from build123d import *

# Parameters (mm, degrees)
EXTRUDE_1_DEPTH = 2


with BuildPart() as part:
    # 草图1 → 凸台-拉伸1 (new body)
    with BuildSketch(Plane.XY):
        with BuildLine():
            Line((-56, 150), (56, 150))
            ThreePointArc((56, 150), (58.828427125, 148.828427125), (60, 146))
            Line((60, 146), (60, 144))
            ThreePointArc((60, 144), (58.828427125, 141.171572875), (56, 140))
            Line((56, 140), (8, 140))
            Line((8, 140), (8, -140))
            Line((8, -140), (56, -140))
            ThreePointArc((56, -140), (58.828427125, -141.171572875), (60, -144))
            Line((60, -144), (60, -146))
            ThreePointArc((60, -146), (58.828427125, -148.828427125), (56, -150))
            Line((56, -150), (-56, -150))
            ThreePointArc((-56, -150), (-58.828427125, -148.828427125), (-60, -146))
            Line((-60, -146), (-60, -144))
            ThreePointArc((-60, -144), (-58.828427125, -141.171572875), (-56, -140))
            Line((-56, -140), (-8, -140))
            Line((-8, -140), (-8, 140))
            Line((-8, 140), (-56, 140))
            ThreePointArc((-56, 140), (-58.828427125, 141.171572875), (-60, 144))
            Line((-60, 144), (-60, 146))
            ThreePointArc((-60, 146), (-58.828427125, 148.828427125), (-56, 150))
        make_face()
    extrude(amount=EXTRUDE_1_DEPTH)


solid = part.part
Geometry: final body of the model. Coordinates: model frame, mm. Give positions to 0.01 mm unless a question says otherwise; leave off trailing zeros. Loops run counter-clockwise (first coordinate to the right, second up) from the corner with the lowest first, then second, coordinate; pieces in that order, holes last. Notation, with made-up numbers: M 33,22.25 L 50,22.25 A25 ccw 50,37.25 Z; hole C -30.5,57 d7. An arc over 180 degrees is marked long. Put each result on its own line as item: value.
1) Material intervals for L1, parallel to Y at x = -25, z = 1.25; L2, parallel to X at y = -133, z = 0.65, sorted ascending. Write a range as from..to.
Computed values:
L1: y = -150..-140, 140..150
L2: x = -8..8
2) Cut plane A-A, the plane x = -17. Return the cut outline in (y, z).
Computed values:
outline: M -150,0 L -140,0 L -140,2 L -150,2 Z; M 140,0 L 150,0 L 150,2 L 140,2 Z
3) Cut plane B-B, the plane z = 1.35. Return the cut outline in (x, y), plus the area to 3 significant figures.
Computed values:
outline: M -60,-146 A4 ccw -56,-150 L 56,-150 A4 ccw 60,-146 L 60,-144 A4 ccw 56,-140 L 8,-140 L 8,140 L 56,140 A4 ccw 60,144 L 60,146 A4 ccw 56,150 L -56,150 A4 ccw -60,146 L -60,144 A4 ccw -56,140 L -8,140 L -8,-140 L -56,-140 A4 ccw -60,-144 Z
area: 6,850 mm^2
4) Cut plane C-C, the plane y = 60.5. Return the cut outline in (x, z).
Computed values:
outline: M -8,0 L 8,0 L 8,2 L -8,2 Z
